from build123d import *

# Parameters (mm, degrees)
EXTRUDE_1_DEPTH     = 15
SKETCH_2_R          = 1.5
EXTRUDE_2_DEPTH     = 5
SKETCH_3_R          = 1.5
CUT_EXTRUDE_1_DEPTH = 5


with BuildPart() as part:
    # 草圖1 → 填料-伸長1 (new body)
    with BuildSketch(Plane(origin=(0, 0, 0), x_dir=(1, 0, 0), z_dir=(0, 1, 0))):
        Polygon((2.886751346, 0), (1.443375673, 2.5), (-1.443375673, 2.5), (-2.886751346, 0), (-1.443375673, -2.5), (1.443375673, -2.5), align=None)
    extrude(amount=EXTRUDE_1_DEPTH)

    # 草圖2 → 填料-伸長2 (add)
    with BuildSketch(Plane(origin=(0, 15, 0), x_dir=(1, 0, 0), z_dir=(0, 1, 0))):
        Circle(SKETCH_2_R)
    extrude(amount=EXTRUDE_2_DEPTH)

    # 草圖3 → 除料-伸長1 (cut)
    with BuildSketch(Plane.XZ):
        Circle(SKETCH_3_R)
    extrude(amount=-CUT_EXTRUDE_1_DEPTH, mode=Mode.SUBTRACT)


solid = part.part
The listing builds one solid part. Answer for the finished solid, in the listing's coordinates (mm). A direction names the side the tool comes from. Round coordinates to 2 decimals unless told otherwise and drop trailing zeros. Order: outer loops, then holes, each group sorted by start corner. A loop starts at its lowest first (then second) coordinate and runs counter-clockwise, first axis right, second up. Notation, with made-up numbers: (57, -31) -> (64, -31) arc R8 cw to (64, -27) -> close; hole circle Ø7 at (37.5, -11.5). An arc over 180 degrees is marked (long way). Write each question's results on one line, items separated by ' | '. Start each with the question number.
Q1. Find section D-D (y = 17.25). Determine the outline of the cut face in (x, z), then the cut area to 3 significant figures.
Q2. The mould has two halves that part along Z. Classify faces 1 (the flat face through (0, 5, 0)), 2 (the flat face through (0, 7, 2.5)), 3 (the flat face through (2.175, 7.395, -1.233)): pulls with the +Z half, pulls with the -Z half, needs draft (parallel to the pull), parting line crosses it, or undercut.
Q3. This flat-tipped pin is pushed along its axis until it touches: pin 1 (2.5 mm diameter, centred on x = 0, z = 0, fed in from -Y). Where does it stop, or does it pass through?
Q4. Which of the six approach directions +Z, -Z, +X, -X, +Y, -Y give full straight-line access (tool end or side, diameter ignored) to faces 4 (the cylindrical face through (-1.5, 17.46, -0.07)), 5 (the flat face through (-2.175, 7.395, 1.233)), 6 (the cylindrical face through (-1.5, 2.46, 0.07))?
Q5. Straight lines are drawn through the part: probe 1 along Z at (x, y) = (0, 3.25); probe 2 along Y at (x, z) = (-0.9, 1.55); probe 3 along Y at (x, z) = (-0.1, -0.3). For each, find the intervals that lie inside material, in ascending order. Write a range as from..to.
Q6. Find section A-A (x = 0). Determine the outline of the cut face in (y, z), then the cut area to 3 significant figures.
Q7. Find section C-C (y = 12). Determine the outline of the cut face in (x, z).
Q8. Find section B-B (z = 1.15). Determine the outline of the cut face in (x, y), then the cut area to 3 significant figures.
Worked answers:
1) outline: circle Ø3 at (0, 0) | area: 7.07 mm2
2) face 1: undercut | face 2: pulls with the +Z half | face 3: pulls with the -Z half
3) pin 1: stops at y = 5
4) face 4: +Y | face 5: +Z, -X, +Y, -Y | face 6: -Y
5) probe 1: z = -2.5..-1.5, 1.5..2.5 | probe 2: y = 0..15 | probe 3: y = 5..20
6) outline: (0, -2.5) -> (15, -2.5) -> (15, -1.5) -> (20, -1.5) -> (20, 1.5) -> (15, 1.5) -> (15, 2.5) -> (0, 2.5) -> (0, 1.5) -> (5, 1.5) -> (5, -1.5) -> (0, -1.5) -> close | area: 75.0 mm2
7) outline: (-2.89, 0) -> (-1.44, -2.5) -> (1.44, -2.5) -> (2.89, 0) -> (1.44, 2.5) -> (-1.44, 2.5) -> close
8) outline: (-2.22, 0) -> (-0.96, 0) -> (-0.96, 5) -> (0.96, 5) -> (0.96, 0) -> (2.22, 0) -> (2.22, 15) -> (0.96, 15) -> (0.96, 20) -> (-0.96, 20) -> (-0.96, 15) -> (-2.22, 15) -> close | area: 66.7 mm2
